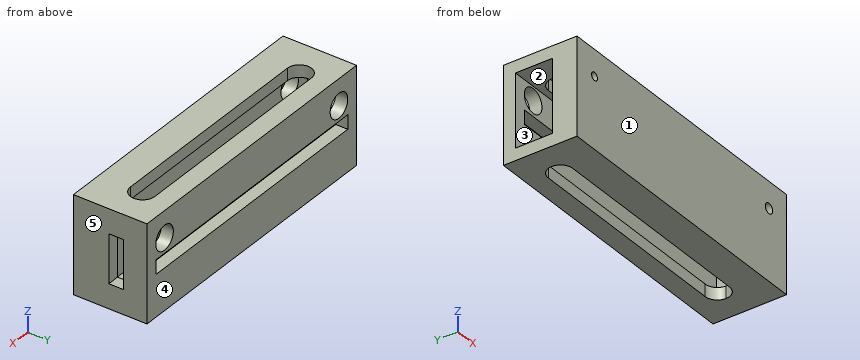
from build123d import *

# Parameters (mm, degrees)
SKETCH1_W            = 65.5
SKETCH1_H            = 9
SKETCH1_R            = 0.998395378
SKETCH1_R_2          = 1.243115981
BOSS_EXTRUDE1_DEPTH  = 6
SKETCH3_W            = 65.5
SKETCH3_H            = 6
BOSS_EXTRUDE2_DEPTH  = 10
SKETCH4_W            = 65.5
SKETCH4_H            = 6
BOSS_EXTRUDE3_DEPTH  = 2
SKETCH5_W            = 65.5
SKETCH5_H            = 3
BOSS_EXTRUDE4_DEPTH  = 9.2
SKETCH7_W            = 21
SKETCH7_H            = 15.2
BOSS_EXTRUDE6_DEPTH  = 3
SKETCH12_W           = 68.5
SKETCH12_H           = 15.2
BOSS_EXTRUDE10_DEPTH = 3
SKETCH13_W           = 24
SKETCH13_H           = 15.2
SKETCH13_W_2         = 12
SKETCH13_H_2         = 3.7
BOSS_EXTRUDE11_DEPTH = 3
CUT_EXTRUDE2_DEPTH   = 25
SKETCH11_W           = 18
SKETCH11_H           = 9.2
CUT_EXTRUDE4_DEPTH   = 3
SKETCH14_W           = 71.5
SKETCH14_H           = 24
BOSS_EXTRUDE12_DEPTH = 3
SKETCH15_W           = 65.5
SKETCH15_H           = 3.5
CUT_EXTRUDE5_DEPTH   = 3
SKETCH16_R           = 3
CUT_EXTRUDE6_DEPTH   = 15.2


with BuildPart() as part:
    # Sketch1 → Boss-Extrude1 (new body)
    with BuildSketch(Plane(origin=(0, 0, 0), x_dir=(1, 0, 0), z_dir=(0, 1, 0))):
        Rectangle(SKETCH1_W, SKETCH1_H)
        with Locations((-29.75, 0)):
            Circle(SKETCH1_R, mode=Mode.SUBTRACT)
        with Locations((29.75, 0)):
            Circle(SKETCH1_R_2, mode=Mode.SUBTRACT)
    extrude(amount=BOSS_EXTRUDE1_DEPTH)

    # Sketch3 → Boss-Extrude2 (add)
    with BuildSketch(Plane(origin=(0, 0, -4.5), x_dir=(-1, 0, 0), z_dir=(0, 0, -1))):
        with Locations((0, 3)):
            Rectangle(SKETCH3_W, SKETCH3_H)
    extrude(amount=BOSS_EXTRUDE2_DEPTH)

    # Sketch4 → Boss-Extrude3 (add)
    with BuildSketch(Plane.XY.offset(4.5)):
        with Locations((0, 3)):
            Rectangle(SKETCH4_W, SKETCH4_H)
    extrude(amount=BOSS_EXTRUDE3_DEPTH)

    # Sketch5 → Boss-Extrude4 (add)
    with BuildSketch(Plane(origin=(0, 6, 0), x_dir=(1, 0, 0), z_dir=(0, 1, 0))):
        with Locations((0, -5)):
            Rectangle(SKETCH5_W, SKETCH5_H)
    extrude(amount=BOSS_EXTRUDE4_DEPTH)

    # Sketch7 → Boss-Extrude6 (add)
    with BuildSketch(Plane.ZY.offset(32.75)):
        with Locations((-4, 7.6)):
            Rectangle(SKETCH7_W, SKETCH7_H)
    extrude(amount=BOSS_EXTRUDE6_DEPTH)

    # Sketch12 → Boss-Extrude10 (add)
    with BuildSketch(Plane(origin=(0, 0, -14.5), x_dir=(-1, 0, 0), z_dir=(0, 0, -1))):
        with Locations((1.5, 7.6)):
            Rectangle(SKETCH12_W, SKETCH12_H)
    extrude(amount=BOSS_EXTRUDE10_DEPTH)

    # Sketch13 → Boss-Extrude11 (add)
    with BuildSketch(Plane(origin=(32.75, 0, 0), x_dir=(0, 0, -1), z_dir=(1, 0, 0))):
        with Locations((5.5, 7.6)):
            Rectangle(SKETCH13_W, SKETCH13_H)
        with Locations((5.5, 10.6)):
            Rectangle(SKETCH13_W_2, SKETCH13_H_2, mode=Mode.SUBTRACT)
    extrude(amount=BOSS_EXTRUDE11_DEPTH)

    # Sketch6 → Cut-Extrude2 (cut, through all)
    with BuildSketch(Plane.XY.offset(6.5)):
        with BuildLine():
            ThreePointArc((-23.75, 10.6), (-24.628679656, 12.721320344), (-26.75, 13.6))
            Line((-26.75, 13.6), (-26.75, 7.6))
            ThreePointArc((-26.75, 7.6), (-24.628679656, 8.478679656), (-23.75, 10.6))
        make_face()
        with BuildLine():
            Line((-26.75, 7.6), (-26.75, 13.6))
            ThreePointArc((-26.75, 13.6), (-29.75, 10.6), (-26.75, 7.6))
        make_face()
        with BuildLine():
            ThreePointArc((29.75, 10.6), (28.871320344, 12.721320344), (26.75, 13.6))
            Line((26.75, 13.6), (26.75, 7.6))
            ThreePointArc((26.75, 7.6), (28.871320344, 8.478679656), (29.75, 10.6))
        make_face()
        with BuildLine():
            Line((26.75, 7.6), (26.75, 13.6))
            ThreePointArc((26.75, 13.6), (23.75, 10.6), (26.75, 7.6))
        make_face()
        with BuildLine():
            Line((26.75, 13.6), (-26.75, 13.6))
            ThreePointArc((-26.75, 13.6), (-24.628679656, 12.721320344), (-23.75, 10.6))
            ThreePointArc((-23.75, 10.6), (-24.628679656, 8.478679656), (-26.75, 7.6))
            Line((-26.75, 7.6), (26.75, 7.6))
            ThreePointArc((26.75, 7.6), (23.75, 10.6), (26.75, 13.6))
        make_face()
    extrude(amount=-CUT_EXTRUDE2_DEPTH, mode=Mode.SUBTRACT)

    # Sketch11 → Cut-Extrude4 (cut)
    with BuildSketch(Plane.ZY.offset(35.75)):
        with Locations((-5.5, 10.6)):
            Rectangle(SKETCH11_W, SKETCH11_H)
    extrude(amount=-CUT_EXTRUDE4_DEPTH, mode=Mode.SUBTRACT)

    # Sketch14 → Boss-Extrude12 (add)
    with BuildSketch(Plane(origin=(0, 15.2, 0), x_dir=(1, 0, 0), z_dir=(0, 1, 0))):
        with Locations((0, 5.5)):
            Rectangle(SKETCH14_W, SKETCH14_H)
    extrude(amount=BOSS_EXTRUDE12_DEPTH)

    # Sketch15 → Cut-Extrude5 (cut)
    with BuildSketch(Plane(origin=(0, 18.2, 0), x_dir=(1, 0, 0), z_dir=(0, 1, 0))):
        with Locations((0, 5.5)):
            Rectangle(SKETCH15_W, SKETCH15_H)
    extrude(amount=-CUT_EXTRUDE5_DEPTH, mode=Mode.SUBTRACT)

    # Sketch16 → Cut-Extrude6 (cut)
    with BuildSketch(Plane(origin=(0, 18.2, 0), x_dir=(1, 0, 0), z_dir=(0, 1, 0))):
        with Locations((-29.75, 0)):
            Circle(SKETCH16_R)
        with Locations((29.75, 0)):
            Circle(SKETCH16_R)
    extrude(amount=-CUT_EXTRUDE6_DEPTH, mode=Mode.SUBTRACT)


solid = part.part
The model under review builds one solid part; all positions refer to its coordinate system, in mm. Face numbers are marked on the shaded views. A direction names the side the tool comes from. Give positions to 0.01 mm unless a question says otherwise; leave off trailing zeros. Loops run counter-clockwise (first coordinate to the right, second up) from the corner with the lowest first, then second, coordinate; pieces in that order, holes last. Notation, with made-up numbers: (14, 2.5) -> (53, 2.5) arc R16 ccw to (53, 11.5) -> close; hole circle Ø2 at (-30.75, 77). An arc over 180 degrees is marked (long way). Answer as a JSON object with one key per item and string values. Group by question number.
Q1. Draft analysis for pull direction Y (two halves, no side actions). For the marked faces 3, 4 and 5, state which applies: pulls with the +Y half, pulls with the -Y half, needs draft (parallel to the pull), parting line crosses it, or undercut.
Q2. Take a section at C-C (z = -12.25). Write out the cut boundary in (x, y).
Q3. Take a section at B-B (z = 4.75). Write out the cut boundary in (x, y), plus the area to 3 significant figures.
Q4. Insertion check: pin 1 (10 mm diameter, centred on x = -16.5, y = 9, fed in from -Z); pin 2 (3.5 mm diameter, centred on y = 11, z = -6.5, fed in from -X); pin 3 (3.5 mm diameter, centred on x = 29.75, z = 0, fed in from +Y). Each pin has a flat end and moves straight along its axis. Give the tip position at first contact, or say it passes through.
Q5. Take a section at D-D (y = 5). Write out the cut boundary in (x, z), plus the area to 3 significant figures.
Q6. Tool access review of the marked faces 1 and 2: name each direction out of +Z, -Z, +X, -X, +Y, -Y from which nothing blocks a thin tool from reaching the whole face with its end or side.
Q7. Wall thickness on line 1 along X through (y, z) = (16.65, 0); line 2 along Z through (x, y) = (29.75, 16.1); line 3 along Y through (x, z) = (20.5, -11): over which ranges is each line inside the solid? List them lowest first.
Q8. Take a section at A-A (x = 11.5). Write out the cut boundary in (y, z).
Answer below:
{
 "1": {"face 3": "undercut", "face 4": "pulls with the +Y half", "face 5": "needs draft"},
 "2": {"outline": "(-35.75, 0) -> (35.75, 0) -> (35.75, 18.2) -> (-35.75, 18.2) -> (-35.75, 15.2) -> (32.75, 15.2) -> (32.75, 6) -> (-35.75, 6) -> close"},
 "3": {"outline": "(-35.75, 0) -> (35.75, 0) -> (35.75, 18.2) -> (-35.75, 18.2) -> close; hole (-26.75, 7.6) -> (26.75, 7.6) arc R3 ccw to (26.75, 13.6) -> (-26.75, 13.6) arc R3 ccw to start", "area": "952 mm2"},
 "4": {"pin 1": "stops at z = -17.5", "pin 2": "stops at x = 32.75", "pin 3": "stops at y = 3"},
 "5": {"outline": "(-35.75, -17.5) -> (35.75, -17.5) -> (35.75, 6.5) -> (-35.75, 6.5) -> close; hole circle Ø6 at (-29.75, 0); hole circle Ø6 at (29.75, 0)", "area": "1,660 mm2"},
 "6": {"face 1": "+Z, -Z, +X, -X, -Y", "face 2": "-X"},
 "7": {"line 1": "x = -35.75 to -32.75, -26.75 to 26.75, 32.75 to 35.75", "line 2": "z = -17.5 to -7.25, -3.75 to -3, 3 to 6.5", "line 3": "y = 0 to 6, 15.2 to 18.2"},
 "8": {"outline": "(0, -17.5) -> (7.6, -17.5) -> (7.6, -14.5) -> (6, -14.5) -> (6, 3.5) -> (7.6, 3.5) -> (7.6, 6.5) -> (0, 6.5) -> close; (13.6, -17.5) -> (18.2, -17.5) -> (18.2, -7.25) -> (15.2, -7.25) -> (15.2, -14.5) -> (13.6, -14.5) -> close; (13.6, 3.5) -> (15.2, 3.5) -> (15.2, -3.75) -> (18.2, -3.75) -> (18.2, 6.5) -> (13.6, 6.5) -> close"}
}
